Answer from the drawing. Dimensions are ordinates in mm from the lowest x, y and z of the part. A direction names the side the tool comes from. Coordinates: 2 decimals unless noted, no trailing zeros. Loops run counter-clockwise (first coordinate to the right, second up) from the corner with the lowest first, then second, coordinate; pieces in that order, holes last. Notation, with made-up numbers: (-27.5, 6) - (12.5, 6) arc R25 cw to (12.5, 20) - close; hole circle Ø6 at (-9.5, 72.25). An arc over 180 degrees is marked (long way). Use one line per item in the form item = value. Start each with the question number.
1) A cutting plane is placed at A-A (z = 31). Give the vertices of the cut face in (x, y), and give its area (3 significant figures).
2) The mould has two halves that part along Y. Classify the marked faces 1, 2, 3 and 4: released by +Y, released by -Y, zero draft, split by the parting line, or undercut.
3) Consider line 1 (Y direction, x = 60, z = 18); line 2 (Y direction, x = 60, z = 36). Determine where each line is inside the solid, lowest interval first.
4) A cutting plane is placed at B-B (x = 60). Give the vertices of the cut face in (y, z), and give its area (3 significant figures).
5) Which of the six approach directions +Z, -Z, +X, -X, +Y, -Y give full straight-line access (tool end or side, diameter ignored) to the marked faces 5, 6 and 7?
6) A cutting plane is placed at D-D (y = 23). Give the vertices of the cut face in (x, z).
7) Each of these flat-tipped pins is pushed along its axis until it touches: P1, Ø8.5, axis at x = 50.5, z = 38, coming from the -Y side; P2, Ø2, axis at x = 32, y = 90.5, coming from the +Z side; P3, Ø4, axis at x = 96, y = 40, coming from the -Z side. Where does it stop, or does it pass through?
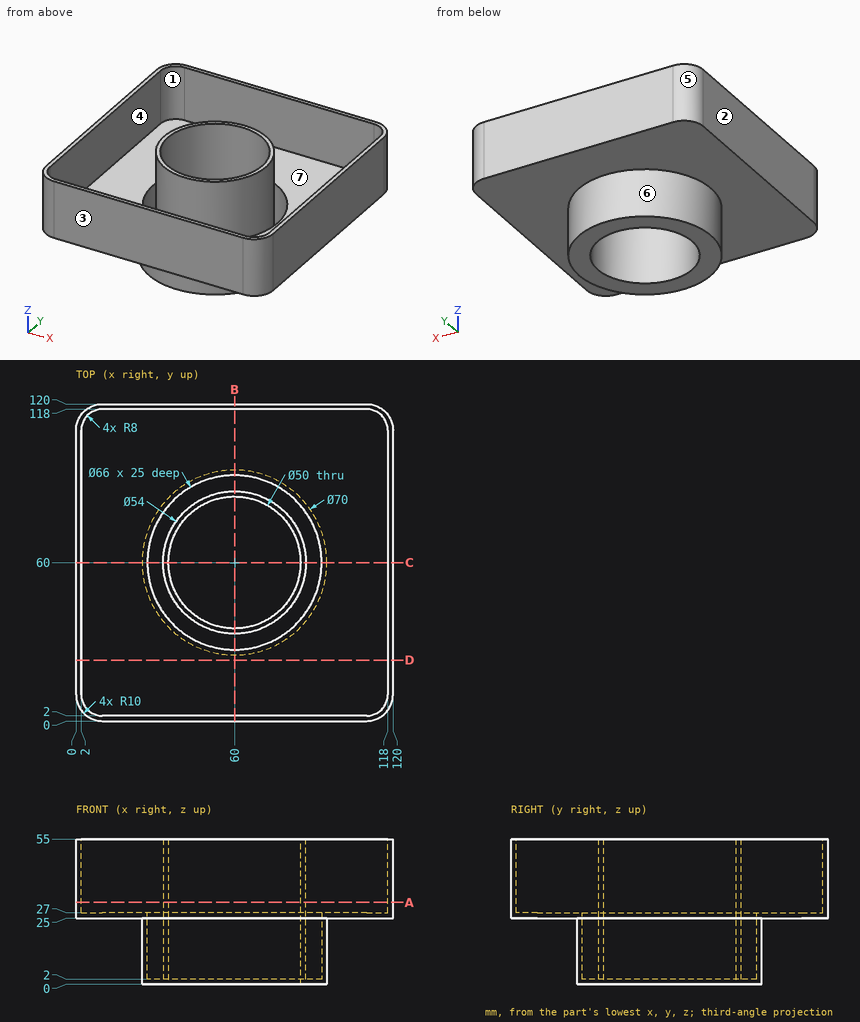
Found:
q1.outline = (0, 10) arc R10 ccw to (10, 0) - (110, 0) arc R10 ccw to (120, 10) - (120, 110) arc R10 ccw to (110, 120) - (10, 120) arc R10 ccw to (0, 110) - close; circle Ø54 at (60, 60); hole (2, 10) arc R8 ccw to (10, 2) - (110, 2) arc R8 ccw to (118, 10) - (118, 110) arc R8 ccw to (110, 118) - (10, 118) arc R8 ccw to (2, 110) - close; hole circle Ø50 at (60, 60)
q1.area = 1,240 mm^2
q2.face_1 = undercut
q2.face_2 = zero draft
q2.face_3 = released by -Y
q2.face_4 = undercut
q3.line_1 = 25 to 27, 33 to 35, 85 to 87, 93 to 95
q3.line_2 = 0 to 2, 33 to 35, 85 to 87, 118 to 120
q4.outline = (0, 25) - (25, 25) - (25, 0) - (35, 0) - (35, 55) - (33, 55) - (33, 2) - (27, 2) - (27, 27) - (2, 27) - (2, 55) - (0, 55) - close; (85, 0) - (95, 0) - (95, 25) - (120, 25) - (120, 55) - (118, 55) - (118, 27) - (93, 27) - (93, 2) - (87, 2) - (87, 55) - (85, 55) - close
q4.area = 564 mm^2
q5.face_5 = +Z, -Z, -X, +Y
q5.face_6 = -Z
q5.face_7 = +Z
q6.outline = (0, 25) - (120, 25) - (120, 55) - (118, 55) - (118, 27) - (2, 27) - (2, 55) - (0, 55) - close
q7.P1 = 0
q7.P2 = 27
q7.P3 = 25
